from build123d import *

# Parameters (mm, degrees)
SKETCH_1_W               = 28
SKETCH_1_H               = 20.3
SKETCH_1_R               = 1.5
EXTRUDE_1_DEPTH          = 5
SKETCH_2_W               = 28
SKETCH_2_H               = 6
SKETCH_2_H_2             = 4
EXTRUDE_2_DEPTH          = 10
SKETCH_3_W               = 28
SKETCH_3_H               = 6
EXTRUDE_3_DEPTH          = 5
SKETCH_4_R               = 1.5
CUT_EXTRUDE_1_DEPTH      = 27.11173108
SKETCH_5_W               = 10
SKETCH_5_H               = 6
SKETCH_5_W_2             = 5
SKETCH_5_H_2             = 4
CUT_EXTRUDE_2_DEPTH      = 34.835225727
SKETCH_6_W               = 28
SKETCH_6_H               = 30.3
CUT_EXTRUDE_3_DEPTH      = 1
EXTRUDE_4_DEPTH          = 12
EXTRUDE_4_DEPTH_BACK     = 10
SKETCH_7_W               = 28
SKETCH_7_H               = 4
CUT_EXTRUDE_4_DEPTH      = 28.313412456
CUT_EXTRUDE_4_DEPTH_BACK = 1.5
SKETCH_9_R               = 3.1
SKETCH_9_R_2             = 1.5
CUT_EXTRUDE_5_DEPTH      = 41.354553646
CUT_EXTRUDE_5_DEPTH_BACK = 41.354553646
SKETCH_10_R              = 1.55
SKETCH_11_W              = 12
SKETCH_11_H              = 30.3
SKETCH_11_W_2            = 6
EXTRUDE_5_DEPTH          = 3
FILLET_1_R               = 2
FILLET_2_R               = 3
EXTRUDE_START            = 2
SKETCH_13_W              = 28
SKETCH_13_H              = 30.3
SKETCH_13_R              = 3.1
EXTRUDE_6_DEPTH          = 2


with BuildPart() as part:
    # 草图1 → 凸台-拉伸1 (new body)
    with BuildSketch(Plane.XY):
        Rectangle(SKETCH_1_W, SKETCH_1_H)
        with Locations((-5, 7.5)):
            Circle(SKETCH_1_R, mode=Mode.SUBTRACT)
        with Locations((5, 7.5)):
            Circle(SKETCH_1_R, mode=Mode.SUBTRACT)
        with Locations((5, -7.5)):
            Circle(SKETCH_1_R, mode=Mode.SUBTRACT)
        with Locations((-5, -7.5)):
            Circle(SKETCH_1_R, mode=Mode.SUBTRACT)
    extrude(amount=EXTRUDE_1_DEPTH)

    # 草图2 → 凸台-拉伸2 (add)
    with BuildSketch(Plane.XY.offset(5)):
        with Locations((0, 13.15)):
            Rectangle(SKETCH_2_W, SKETCH_2_H)
        with Locations((0, -12.15)):
            Rectangle(SKETCH_2_W, SKETCH_2_H_2)
    extrude(amount=-EXTRUDE_2_DEPTH)

    # 草图3 → 凸台-拉伸3 (add)
    with BuildSketch(Plane(origin=(0, 0, -5), x_dir=(-1, 0, 0), z_dir=(0, 0, -1))):
        with Locations((0, 13.15)):
            Rectangle(SKETCH_3_W, SKETCH_3_H)
    extrude(amount=EXTRUDE_3_DEPTH)

    # 草图4 → 切除-拉伸1 (cut, through all)
    with BuildSketch(Plane.XY.offset(5)):
        with Locations((-9, 13.15)):
            Circle(SKETCH_4_R)
        with Locations((9, 13.15)):
            Circle(SKETCH_4_R)
    extrude(amount=-CUT_EXTRUDE_1_DEPTH, mode=Mode.SUBTRACT)

    # 草图5 → 切除-拉伸2 (cut, through all)
    with BuildSketch(Plane.ZY.offset(14)):
        with Locations((-5, 13.15)):
            Rectangle(SKETCH_5_W, SKETCH_5_H)
        with Locations((-2.5, -12.15)):
            Rectangle(SKETCH_5_W_2, SKETCH_5_H_2)
    extrude(amount=-CUT_EXTRUDE_2_DEPTH, mode=Mode.SUBTRACT)

    # 草图6 → 切除-拉伸3 (cut)
    with BuildSketch(Plane.XY.offset(5)):
        with Locations((0, 1)):
            Rectangle(SKETCH_6_W, SKETCH_6_H)
    extrude(amount=-CUT_EXTRUDE_3_DEPTH, mode=Mode.SUBTRACT)

    # 草图7 → 凸台-拉伸4 (add, two sides: drawn at the far end of the back side and taken through both)
    with BuildSketch(Plane.XY.offset(4).offset(-EXTRUDE_4_DEPTH_BACK)):
        with Locations((0, 18.15)):
            Rectangle(SKETCH_7_W, SKETCH_7_H)
        with Locations((0, -16.15)):
            Rectangle(SKETCH_7_W, SKETCH_7_H)
    extrude(amount=EXTRUDE_4_DEPTH + EXTRUDE_4_DEPTH_BACK)

    # 草图9 → 切除-拉伸4 (cut, two sides: drawn at the far end of the back side and taken through both)
    # profile 1 of 6: a face of its own
    with BuildSketch(Plane.XY.offset(4).offset(-CUT_EXTRUDE_4_DEPTH_BACK)):
        with Locations((-5, 7.5)):
            Circle(SKETCH_9_R)
        with Locations((-5, 7.5)):
            Circle(SKETCH_9_R_2, mode=Mode.SUBTRACT)
    # profile 2 of 6: a face of its own
    with BuildSketch(Plane.XY.offset(4).offset(-CUT_EXTRUDE_4_DEPTH_BACK)):
        with Locations((5, 7.5)):
            Circle(SKETCH_9_R)
        with Locations((5, 7.5)):
            Circle(SKETCH_9_R_2, mode=Mode.SUBTRACT)
    # profile 3 of 6: a face of its own
    with BuildSketch(Plane.XY.offset(4).offset(-CUT_EXTRUDE_4_DEPTH_BACK)):
        with Locations((5, -7.5)):
            Circle(SKETCH_9_R)
        with Locations((5, -7.5)):
            Circle(SKETCH_9_R_2, mode=Mode.SUBTRACT)
    # profile 4 of 6: a face of its own
    with BuildSketch(Plane.XY.offset(4).offset(-CUT_EXTRUDE_4_DEPTH_BACK)):
        with Locations((-5, -7.5)):
            Circle(SKETCH_9_R)
        with Locations((-5, -7.5)):
            Circle(SKETCH_9_R_2, mode=Mode.SUBTRACT)
    # profile 5 of 6: a face of its own
    with BuildSketch(Plane.XY.offset(4).offset(-CUT_EXTRUDE_4_DEPTH_BACK)):
        Polygon((-7.36898549, 10.325), (-5.737970979, 13.15), (-7.36898549, 15.975), (-10.63101451, 15.975), (-12.262029021, 13.15), (-10.63101451, 10.325), align=None)
        with Locations((-9, 13.15)):
            Circle(SKETCH_9_R_2, mode=Mode.SUBTRACT)
    # profile 6 of 6: a face of its own
    with BuildSketch(Plane.XY.offset(4).offset(-CUT_EXTRUDE_4_DEPTH_BACK)):
        Polygon((10.63101451, 10.325), (12.262029021, 13.15), (10.63101451, 15.975), (7.36898549, 15.975), (5.737970979, 13.15), (7.36898549, 10.325), align=None)
        with Locations((9, 13.15)):
            Circle(SKETCH_9_R_2, mode=Mode.SUBTRACT)
    extrude(amount=CUT_EXTRUDE_4_DEPTH + CUT_EXTRUDE_4_DEPTH_BACK, mode=Mode.SUBTRACT)

    # 草图10 → 切除-拉伸5 (cut, two sides: drawn at the far end of the back side and taken through both)
    with BuildSketch(Plane(origin=(0, -14.15, 0), x_dir=(1, 0, 0), z_dir=(0, 1, 0)).offset(-CUT_EXTRUDE_5_DEPTH_BACK)):
        with Locations(Location((-9, -11, 0), (0, 0, 270))):
            Circle(SKETCH_10_R)
        with Locations(Location((9, -11, 0), (0, 0, 270))):
            Circle(SKETCH_10_R)
    extrude(amount=CUT_EXTRUDE_5_DEPTH + CUT_EXTRUDE_5_DEPTH_BACK, mode=Mode.SUBTRACT)

    # 草图11 → 凸台-拉伸5 (add)
    with BuildSketch(Plane(origin=(14, 0, 0), x_dir=(0, 0, -1), z_dir=(1, 0, 0))):
        Polygon((-16, 16.15), (-4, 16.15), (-4, -14.15), (-16, -14.15), (-16, -18.15), (6, -18.15), (6, -14.15), (0, -14.15), (0, 16.15), (6, 16.15), (6, 20.15), (-16, 20.15), align=None)
        with Locations((-10, 1)):
            Rectangle(SKETCH_11_W, SKETCH_11_H)
        with Locations((3, 1)):
            Rectangle(SKETCH_11_W_2, SKETCH_11_H)
    extrude(amount=EXTRUDE_5_DEPTH)

    # 圆角1
    fillet_1_edges = [part.edges().sort_by_distance(p)[0] for p in [
        (17, 20.15, 5),
        (17, -18.15, 5),
    ]]
    fillet(fillet_1_edges, radius=FILLET_1_R)

    # 圆角2
    fillet_2_edges = [part.edges().sort_by_distance(p)[0] for p in [
        (-14, 18.15, 16),
        (-14, 18.15, -6),
        (-14, -16.15, -6),
        (-14, -16.15, 16),
    ]]
    fillet(fillet_2_edges, radius=FILLET_2_R)

    # 草图13 → 凸台-拉伸6 (add)
    with BuildSketch(Plane.XY.offset(4).offset(EXTRUDE_START)):
        with Locations((0, 1)):
            Rectangle(SKETCH_13_W, SKETCH_13_H)
        with Locations((5, -7.5)):
            Circle(SKETCH_13_R, mode=Mode.SUBTRACT)
        with Locations((-5, -7.5)):
            Circle(SKETCH_13_R, mode=Mode.SUBTRACT)
        with Locations((5, 7.5)):
            Circle(SKETCH_13_R, mode=Mode.SUBTRACT)
        with Locations((-5, 7.5)):
            Circle(SKETCH_13_R, mode=Mode.SUBTRACT)
        Polygon((-10.63101451, 15.975), (-7.36898549, 15.975), (-5.737970979, 13.15), (-7.36898549, 10.325), (-10.63101451, 10.325), (-12.262029021, 13.15), align=None, mode=Mode.SUBTRACT)
        Polygon((10.63101451, 10.325), (7.36898549, 10.325), (5.737970979, 13.15), (7.36898549, 15.975), (10.63101451, 15.975), (12.262029021, 13.15), align=None, mode=Mode.SUBTRACT)
    extrude(amount=-EXTRUDE_6_DEPTH)


solid = part.part
Design review of the part built by this model. Coordinates are the model's own, in mm. A direction names the side the tool comes from. Coordinates: 2 decimals unless noted, no trailing zeros. Order: outer loops, then holes, each group sorted by start corner. A loop starts at its lowest first (then second) coordinate and runs counter-clockwise, first axis right, second up. Notation, with made-up numbers: (79.5, 42.5) -> (111.5, 42.5) arc R6 ccw to (111.5, 50.5) -> close; hole circle Ø5 at (65.5, 50.25). An arc over 180 degrees is marked (long way). Use one line per item in the form item = value. Start each with the question number.
(1) Add section C-C on y = 7.5. State the section outline as (x, z) points.
(2) The part is to be moulded in two halves that separate along Z. For faces 5 (the flat face through (-14, 1, 3)), 6 (the flat face through (14.3, 1.1, 16)), 7 (the cylindrical face through (-9.94, -16.18, 9.77)), say which applies: +Z half, -Z half, draft (parallel to the pull), parting line (faces both ways), or undercut.
(3) Add section B-B on x = -5. State the section outline as (y, z) points.
(4) For faces 1 (the cylindrical face through (-5, -9, 1)), 2 (the flat face through (4, 6, 2.5)), 3 (the flat face through (0, 16.15, -3)), 4 (the flat face through (0, 1, 6)), list the 3-axis set-ups (+Z, -Z, +X, -X, +Y, -Y) from which the entire face can be reached by the end or side of a thin tool; tool diameter is ignored.
(5) Insertion check: pin 1 (8 mm diameter, centred on y = -5.5, z = 11.5, fed in from -X); pin 2 (7 mm diameter, centred on x = -5, y = -8, fed in from +Z); pin 3 (5 mm diameter, centred on x = 5, y = -7.5, fed in from +Z); pin 4 (2.5 mm diameter, centred on x = -5, y = 7.5, fed in from -Z). Each pin has a flat end and moves straight along its axis. Give the tip position at first contact, or say it passes through.
(6) Add section D-D on x = 9. State the section outline as (y, z) points (3 decimals), plus the area to 3 significant figures.
(7) For probe 1 along X at (y, z) = (-7.5, 4.5); probe 2 along Y at (x, z) = (-5, 3.1); probe 3 along Y at (x, z) = (5, 0.5), list the stretches that pass through material, from the lowest coordinate up.
(8) Add section A-A on z = 11. State the section outline as (x, y) points.
Answer block:
q1.outline = (-14, 0) -> (-6.5, 0) -> (-6.5, 2.5) -> (-8.1, 2.5) -> (-8.1, 6) -> (-14, 6) -> close; (-3.5, 0) -> (3.5, 0) -> (3.5, 2.5) -> (1.9, 2.5) -> (1.9, 6) -> (-1.9, 6) -> (-1.9, 2.5) -> (-3.5, 2.5) -> close; (6.5, 0) -> (14, 0) -> (14, -6) -> (17, -6) -> (17, 16) -> (14, 16) -> (14, 6) -> (8.1, 6) -> (8.1, 2.5) -> (6.5, 2.5) -> close
q2.face_5 = draft
q2.face_6 = +Z half
q2.face_7 = undercut
q3.outline = (-18.15, -6) -> (-14.15, -6) -> (-14.15, 0) -> (-9, 0) -> (-9, 2.5) -> (-10.6, 2.5) -> (-10.6, 6) -> (-14.15, 6) -> (-14.15, 16) -> (-18.15, 16) -> close; (-6, 0) -> (6, 0) -> (6, 2.5) -> (4.4, 2.5) -> (4.4, 6) -> (-4.4, 6) -> (-4.4, 2.5) -> (-6, 2.5) -> close; (9, 0) -> (16.15, 0) -> (16.15, -6) -> (20.15, -6) -> (20.15, 16) -> (16.15, 16) -> (16.15, 6) -> (10.6, 6) -> (10.6, 2.5) -> (9, 2.5) -> close
q4.face_1 = +Z, -Z
q4.face_2 = +Z
q4.face_3 = -Z, -X
q4.face_4 = +Z, -X
q5.pin_1 = 14
q5.pin_2 = 6
q5.pin_3 = 2.5
q5.pin_4 = through
q6.outline = (-18.15, -6) -> (-14.15, -6) -> (-14.15, 0) -> (11.65, 0) -> (11.65, 2.5) -> (10.325, 2.5) -> (10.325, 6) -> (-14.15, 6) -> (-14.15, 9.45) -> (-18.15, 9.45) -> close; (-18.15, 12.55) -> (-14.15, 12.55) -> (-14.15, 16) -> (-18.15, 16) -> close; (14.65, 0) -> (16.15, 0) -> (16.15, -6) -> (20.15, -6) -> (20.15, 9.45) -> (16.15, 9.45) -> (16.15, 6) -> (15.975, 6) -> (15.975, 2.5) -> (14.65, 2.5) -> close; (16.15, 12.55) -> (20.15, 12.55) -> (20.15, 16) -> (16.15, 16) -> close
q6.area = 306 mm²
q7.probe_1 = -14 to -8.1, -1.9 to 1.9, 8.1 to 17
q7.probe_2 = -18.15 to -10.6, -4.4 to 4.4, 10.6 to 20.15
q7.probe_3 = -18.15 to -9, -6 to 6, 9 to 20.15
q8.outline = (-14, -18.15) -> (-10.55, -18.15) -> (-10.55, -14.15) -> (-14, -14.15) -> close; (-14, 16.15) -> (-10.55, 16.15) -> (-10.55, 20.15) -> (-14, 20.15) -> close; (-7.45, -18.15) -> (7.45, -18.15) -> (7.45, -14.15) -> (-7.45, -14.15) -> close; (-7.45, 16.15) -> (7.45, 16.15) -> (7.45, 20.15) -> (-7.45, 20.15) -> close; (10.55, -18.15) -> (15, -18.15) arc R2 ccw to (17, -16.15) -> (17, 18.15) arc R2 ccw to (15, 20.15) -> (10.55, 20.15) -> (10.55, 16.15) -> (14, 16.15) -> (14, -14.15) -> (10.55, -14.15) -> close
